CAD build for the part. Positions are in the model's coordinates, mm. Coordinates: 2 decimals unless noted, no trailing zeros. Write each loop counter-clockwise with the first axis right and the second up, starting at its lowest first coordinate (ties: lowest second). Pieces come first, ordered by that corner, then holes. Notation, with made-up numbers: M -39.5,85 L -28.5,85 A6 cw -28.5,91 Z; hole C 3,59.25 d10. An arc over 180 degrees is marked long. Put each result on its own line as item: value. Start each with the question number.
```python
from build123d import *

# Parameters (mm, degrees)
ESQUISSE1_R             = 5
BOSS_EXTRU_2_DEPTH      = 70
ESQUISSE2_R             = 3.5
BOSS_EXTRU_3_DEPTH      = 12
ESQUISSE4_R             = 15
BOSS_EXTRU_5_DEPTH      = 5
ESQUISSE5_R             = 3.5
BOSS_EXTRU_6_DEPTH      = 12
ENL_V_MAT_EXTRU_1_DEPTH = 12


with BuildPart() as part:
    # Esquisse1 → Boss.-Extru.2 (new body)
    with BuildSketch(Plane.XY):
        Circle(ESQUISSE1_R)
    extrude(amount=BOSS_EXTRU_2_DEPTH)

    # Esquisse2 → Boss.-Extru.3 (add)
    with BuildSketch(Plane(origin=(0, 0, 0), x_dir=(-1, 0, 0), z_dir=(0, 0, -1))):
        Circle(ESQUISSE2_R)
    extrude(amount=BOSS_EXTRU_3_DEPTH)

    # Esquisse4 → Boss.-Extru.5 (add)
    with BuildSketch(Plane.XY.offset(70)):
        Circle(ESQUISSE4_R)
    extrude(amount=-BOSS_EXTRU_5_DEPTH)

    # Esquisse5 → Boss.-Extru.6 (add)
    with BuildSketch(Plane.XY.offset(70)):
        Circle(ESQUISSE5_R)
    extrude(amount=BOSS_EXTRU_6_DEPTH)

    # Esquisse6 → Enlèv. mat.-Extru.1 (cut)
    with BuildSketch(Plane.XY.offset(70)):
        with BuildLine():
            Line((-6.262893089, 8.172072336), (-7.499435292, 12.990707074))
            ThreePointArc((-7.499435292, 12.990707074), (-9.123657799, 11.90625333), (-10.593218546, 10.619968024))
            Line((-10.593218546, 10.619968024), (-6.262893089, 8.172072336))
        make_face()
        with BuildLine():
            Line((-8.152402023, 6.270263162), (-10.606442664, 10.606760769))
            ThreePointArc((-10.606442664, 10.606760769), (-11.894621233, 9.138817524), (-12.981158937, 7.515950549))
            Line((-12.981158937, 7.515950549), (-8.152402023, 6.270263162))
        make_face()
        with BuildLine():
            Line((-9.499942261, 3.951679007), (-12.981158937, 7.515950549))
            ThreePointArc((-12.981158937, 7.515950549), (-13.849269023, 5.761748652), (-14.481582106, 3.909447494))
            Line((-14.481582106, 3.909447494), (-9.499942261, 3.951679007))
        make_face()
        with BuildLine():
            Line((-10.188028074, 1.356459322), (-14.486441985, 3.891400598))
            ThreePointArc((-14.486441985, 3.891400598), (-14.869805294, 1.972027008), (-14.999987869, 0.0190767))
            Line((-14.999987869, 0.0190767), (-10.188028074, 1.356459322))
        make_face()
        with BuildLine():
            ThreePointArc((-14.999987869, -0.0190767), (-14.869805294, -1.972027008), (-14.486441985, -3.891400598))
            Line((-14.486441985, -3.891400598), (-10.188028074, -1.356459322))
            Line((-10.188028074, -1.356459322), (-14.999987869, -0.0190767))
        make_face()
        with BuildLine():
            Line((-9.499942261, -3.951679007), (-14.481582106, -3.909447494))
            ThreePointArc((-14.481582106, -3.909447494), (-13.849269023, -5.761748652), (-12.981158937, -7.515950549))
            Line((-12.981158937, -7.515950549), (-9.499942261, -3.951679007))
        make_face()
        with BuildLine():
            Line((-8.152402023, -6.270263162), (-12.981158937, -7.515950549))
            ThreePointArc((-12.981158937, -7.515950549), (-11.894621233, -9.138817524), (-10.606442664, -10.606760769))
            Line((-10.606442664, -10.606760769), (-8.152402023, -6.270263162))
        make_face()
        with BuildLine():
            Line((-6.262893089, -8.172072336), (-10.593218546, -10.619968024))
            ThreePointArc((-10.593218546, -10.619968024), (-9.123657799, -11.90625333), (-7.499435292, -12.990707074))
            Line((-7.499435292, -12.990707074), (-6.262893089, -8.172072336))
        make_face()
        with BuildLine():
            Line((-3.939593974, -9.504960245), (-7.499435292, -12.990707074))
            ThreePointArc((-7.499435292, -12.990707074), (-5.744130769, -13.8565855), (-3.891026946, -14.486542352))
            Line((-3.891026946, -14.486542352), (-3.939593974, -9.504960245))
        make_face()
        with BuildLine():
            Line((-1.343501295, -10.189744953), (-3.872973884, -14.491379275))
            ThreePointArc((-3.872973884, -14.491379275), (-1.953114292, -14.872301253), (0, -15))
            Line((0, -15), (-1.343501295, -10.189744953))
        make_face()
        with BuildLine():
            ThreePointArc((0, -15), (1.953114292, -14.872301253), (3.872973884, -14.491379275))
            Line((3.872973884, -14.491379275), (1.343501295, -10.189744953))
            Line((1.343501295, -10.189744953), (0, -15))
        make_face()
        with BuildLine():
            ThreePointArc((3.891026946, -14.486542352), (5.744130769, -13.8565855), (7.499435292, -12.990707074))
            Line((7.499435292, -12.990707074), (3.939593974, -9.504960245))
            Line((3.939593974, -9.504960245), (3.891026946, -14.486542352))
        make_face()
        with BuildLine():
            ThreePointArc((7.499435292, -12.990707074), (9.123657799, -11.90625333), (10.593218546, -10.619968024))
            Line((10.593218546, -10.619968024), (6.262893089, -8.172072336))
            Line((6.262893089, -8.172072336), (7.499435292, -12.990707074))
        make_face()
        with BuildLine():
            ThreePointArc((10.606442664, -10.606760769), (11.894621233, -9.138817524), (12.981158937, -7.515950549))
            Line((12.981158937, -7.515950549), (8.152402023, -6.270263162))
            Line((8.152402023, -6.270263162), (10.606442664, -10.606760769))
        make_face()
        with BuildLine():
            ThreePointArc((12.981158937, -7.515950549), (13.849269023, -5.761748652), (14.481582106, -3.909447494))
            Line((14.481582106, -3.909447494), (9.499942261, -3.951679007))
            Line((9.499942261, -3.951679007), (12.981158937, -7.515950549))
        make_face()
        with BuildLine():
            ThreePointArc((15, 0), (14.999996967, 0.009538352), (14.999987869, 0.0190767))
            Line((14.999987869, 0.0190767), (10.159352957, -1.339548494))
            Line((10.159352957, -1.339548494), (14.486441985, -3.891400598))
            ThreePointArc((14.486441985, -3.891400598), (14.87105628, -1.962571047), (15, 0))
        make_face()
        with BuildLine():
            ThreePointArc((14.999987869, 0.0190767), (14.869805294, 1.972027008), (14.486441985, 3.891400598))
            Line((14.486441985, 3.891400598), (10.188028074, 1.356459322))
            Line((10.188028074, 1.356459322), (14.999987869, 0.0190767))
        make_face()
        with BuildLine():
            ThreePointArc((14.481582106, 3.909447494), (13.849269023, 5.761748652), (12.981158937, 7.515950549))
            Line((12.981158937, 7.515950549), (9.499942261, 3.951679007))
            Line((9.499942261, 3.951679007), (14.481582106, 3.909447494))
        make_face()
        with BuildLine():
            ThreePointArc((12.981158937, 7.515950549), (11.894621233, 9.138817524), (10.606442664, 10.606760769))
            Line((10.606442664, 10.606760769), (8.152402023, 6.270263162))
            Line((8.152402023, 6.270263162), (12.981158937, 7.515950549))
        make_face()
        with BuildLine():
            ThreePointArc((10.593218546, 10.619968024), (9.123657799, 11.90625333), (7.499435292, 12.990707074))
            Line((7.499435292, 12.990707074), (6.262893089, 8.172072336))
            Line((6.262893089, 8.172072336), (10.593218546, 10.619968024))
        make_face()
        with BuildLine():
            ThreePointArc((7.499435292, 12.990707074), (5.744130769, 13.8565855), (3.891026946, 14.486542352))
            Line((3.891026946, 14.486542352), (3.939593974, 9.504960245))
            Line((3.939593974, 9.504960245), (7.499435292, 12.990707074))
        make_face()
        with BuildLine():
            ThreePointArc((3.872973884, 14.491379275), (1.953114292, 14.872301253), (0, 15))
            Line((0, 15), (1.343501295, 10.189744953))
            Line((1.343501295, 10.189744953), (3.872973884, 14.491379275))
        make_face()
        with BuildLine():
            Line((-1.343501295, 10.189744953), (0, 15))
            ThreePointArc((0, 15), (-1.953114292, 14.872301253), (-3.872973884, 14.491379275))
            Line((-3.872973884, 14.491379275), (-1.343501295, 10.189744953))
        make_face()
        with BuildLine():
            Line((-3.939593974, 9.504960245), (-3.891026946, 14.486542352))
            ThreePointArc((-3.891026946, 14.486542352), (-5.744130769, 13.8565855), (-7.499435292, 12.990707074))
            Line((-7.499435292, 12.990707074), (-3.939593974, 9.504960245))
        make_face()
    extrude(amount=-ENL_V_MAT_EXTRU_1_DEPTH, mode=Mode.SUBTRACT)


solid = part.part
```
(1) Drill centre lines: line 1 (Z direction, x = 5.5, y = 5.5); line 2 (X direction, y = 12.75, z = 69.5); line 3 (X direction, y = -4.5, z = 45). Where is each one in solid material? Low to high. Write a range as [from, to].
(2) Drop flat-ended pins along their axis: pin 1 (4 mm diameter, centred on x = -2, y = 7, fed in from -Z); pin 2 (2 mm diameter, centred on y = 1.5, z = 27, fed in from +X); pin 3 (4 mm diameter, centred on x = 5.5, y = 3, fed in from -Z); pin 4 (15 mm diameter, centred on x = -0.5, y = 5.5, fed in from -Z). Give the stop position or say it passes through.
(3) Slice it at A-A, the plane x = 12. Write the cut outline in (y, z).
(4) Two-plate mould, pull along X, no slides. Class faces 1 (the face through (-5.69, -11.22, 67.54)), 2 (the face through (-4, 4, 65)), 3 (the face through (-10.533, -6.884, 67.535)): +X half, -X half, draft (parallel to the pull), parting line (faces both ways), or undercut.
Result set:
1. line 1: z = [65, 70]
1. line 2: x = [-7.44, -7.25], [-3.91, -2.85], [-0.63, 0.63], [2.85, 3.91], [7.25, 7.44]
1. line 3: x = [-2.18, 2.18]
2. pin 1: stops at z = 65
2. pin 2: stops at x = 4.97
2. pin 3: stops at z = 0
2. pin 4: stops at z = -12
3. outline: M -7.26,65 L -6.51,65 L -6.51,70 L -7.26,70 Z; M -3.93,65 L -2.43,65 L -2.43,70 L -3.93,70 Z; M -0.82,65 L 0.85,65 L 0.85,70 L -0.82,70 Z; M 2.43,65 L 3.93,65 L 3.93,70 L 2.43,70 Z; M 6.51,65 L 7.26,65 L 7.26,70 L 6.51,70 Z
4. face 1: undercut
4. face 2: draft
4. face 3: undercut
